Geometry: final body of the model. Coordinates: model frame, mm. Face numbers are marked on the shaded views. A direction names the side the tool comes from. Give positions to 0.01 mm unless a question says otherwise; leave off trailing zeros. Loops run counter-clockwise (first coordinate to the right, second up) from the corner with the lowest first, then second, coordinate; pieces in that order, holes last. Notation, with made-up numbers: (-10, -17) -> (35, -17) arc R21 ccw to (35, 5) -> close; hole circle Ø4 at (-33.75, -18). An arc over 180 degrees is marked (long way). One line per item, written item: value. Start each with the question number.
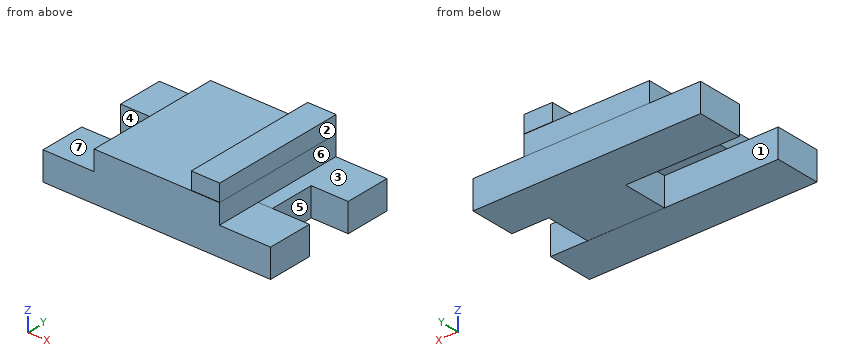
from build123d import *

# Parameters (mm, degrees)
F1_DEPTH      = 69.85
F1_DEPTH_BACK = 69.85
F0_W          = 50.8
F0_H          = 31.75
F2_DEPTH      = 85.725
F3_DEPTH      = 127
F3_DEPTH_BACK = 127
F4_W          = 31.75
F4_H          = 19.05
F5_DEPTH      = 88.9
F5_DEPTH_BACK = 63.5


with BuildPart() as f1:
    # F0 (on Right) → F1 (new body, two sides)
    with BuildSketch(Plane.YZ) as f1_sk:
        Polygon((-89.356257, 22.225), (-89.356257, 0), (-38.556257, 0), (-38.529839, 0), (12.270161, 0), (63.043743, 0), (63.043743, 22.225), (31.293743, 22.225), (-57.606257, 22.225), align=None)
    extrude(amount=F1_DEPTH)
    extrude(f1_sk.sketch, amount=-F1_DEPTH_BACK)

    # F0 (on Right) → F2 (join)
    with BuildSketch(Plane.YZ):
        with Locations((-13.129839, -15.875)):
            Rectangle(F0_W, F0_H)
    extrude(amount=F2_DEPTH)

    # F0 (on Right) → F3 (join, two sides)
    with BuildSketch(Plane.YZ) as f3_sk:
        with Locations((-63.956257, -15.875)):
            Rectangle(F0_W, F0_H)
        Polygon((63.043743, 0), (12.270161, 0), (12.270161, -31.75), (63.070161, -31.75), (63.070161, 0), align=None)
    extrude(amount=F3_DEPTH)
    extrude(f3_sk.sketch, amount=-F3_DEPTH_BACK)

    # F4 (on Front) → F5 (join, two sides)
    with BuildSketch(Plane.XZ) as f5_sk:
        with Locations((53.98327, 31.68009)):
            Rectangle(F4_W, F4_H)
    extrude(amount=F5_DEPTH)
    extrude(f5_sk.sketch, amount=-F5_DEPTH_BACK)


solid = f1.part
Item 1: Section C-C, the plane y = -61. Output: boundary loops of the cut face in (x, z) (3 decimals), then the cut area to 3 significant figures.
Item 2: Mould query, pull axis Z, two halves, no side actions, for the marked faces 1, 2 and 3. Classes: pulls with the +Z half, pulls with the -Z half, needs draft (parallel to the pull), parting line crosses it, or undercut.
Item 3: Access query for the marked faces 4, 5, 6 and 7. Directions: +Z, -Z, +X, -X, +Y, -Y. A direction counts if a zero-diameter tool reaches every point of the face in a straight line with its end or side. Return the directions, or none.
Item 4: Section D-D, the plane x = 8.5. Output: boundary loops of the cut face in (y, z) (3 decimals), then the cut area to 3 significant figures.
Item 5: Ray query, line 1 along Z through (x, y) = (84.5, -71); line 2 along X through (y, z) = (6, -6) (3 decimals); line 3 along Y through (x, z) = (-50.5, -23). Return the intervals inside material, ascending. Write a range as [from, to].
Item 6: Section B-B, the plane z = -10. Output: boundary loops of the cut face in (x, y) (3 decimals).
Item 7: Pin query (flat end, axial travel): pin 1 (15 mm diameter, centred on y = 22.5, z = 29.5, fed in from -X); pin 2 (9.5 mm diameter, centred on x = -0.5, z = -12, fed in from +Y); pin 3 (21 mm diameter, centred on x = 50.5, z = 33.5, fed in from -Y). Return the tip coordinate at first contact, or that it passes through.
Item 8: Section A-A, the plane x = -85. Output: boundary loops of the cut face in (y, z).
Geometry check:
1. outline: (-127, -31.75) -> (127, -31.75) -> (127, 0) -> (69.85, 0) -> (69.85, 22.155) -> (69.858, 22.155) -> (69.858, 41.205) -> (38.108, 41.205) -> (38.108, 22.225) -> (-69.85, 22.225) -> (-69.85, 0) -> (-127, 0) -> close
1. area: 11,800 mm2
2. face 1: undercut
2. face 2: needs draft
2. face 3: pulls with the +Z half
3. face 4: -Z, -X
3. face 5: +Z, -Z, +X
3. face 6: +Z, +X, +Y, -Y
3. face 7: +Z, -X, +Y, -Y
4. outline: (-89.356, -31.75) -> (-38.556, -31.75) -> (-38.556, 0) -> (-38.53, 0) -> (-38.53, -31.75) -> (63.07, -31.75) -> (63.07, 0) -> (63.044, 0) -> (63.044, 22.225) -> (-89.356, 22.225) -> close
4. area: 8,230 mm2
5. line 1: z = [-31.75, 0]
5. line 2: x = [0, 85.725]
5. line 3: y = [-89.36, -38.56], [12.27, 63.07]
6. outline: (-127, -89.356) -> (127, -89.356) -> (127, -38.556) -> (-127, -38.556) -> close; (-127, 12.27) -> (0, 12.27) -> (0, -38.53) -> (85.725, -38.53) -> (85.725, 12.27) -> (127, 12.27) -> (127, 63.07) -> (-127, 63.07) -> close
7. pin 1: stops at x = -69.85
7. pin 2: stops at y = 63.07
7. pin 3: stops at y = -88.9
8. outline: (-89.36, -31.75) -> (-38.56, -31.75) -> (-38.56, 0) -> (-89.36, 0) -> close; (12.27, -31.75) -> (63.07, -31.75) -> (63.07, 0) -> (12.27, 0) -> close
